The model under review builds one solid part; all positions refer to its coordinate system, in mm. Round coordinates to 2 decimals unless told otherwise and drop trailing zeros. Loops run counter-clockwise (first coordinate to the right, second up) from the corner with the lowest first, then second, coordinate; pieces in that order, holes last. Notation, with made-up numbers: M -38,63.5 L 10,63.5 A34 ccw 10,101.5 Z; hole C 29,67.5 d11. An arc over 180 degrees is marked long. Return JSON: item names as keys, results as strings. Group by question number.
Q1. Clearance check with a flat-ended pin moving along its axis: pin 1 Ø7 at (x, y) = (8.255, 17.78) entering from +Z. State where the tip first meets the part, or that it passes through.
Q2. To check wall thickness, follow line 1 along Y through (x, z) = (7, 0.45); line 2 along Y through (x, z) = (8.5, 0.75); line 3 along X through (y, z) = (16.5, 0.45). State the ranges of each line that lie inside material, in increasing order.
Q3. Consider section A-A (z = 0.75). State the section outline as (x, y) points (3 decimals), and give its area (3 significant figures).
Q4. Consider section D-D (x = 22). State the section outline as (y, z) points.
Q5. Draft analysis for pull direction Y (two halves, no side actions). For faces 1 (the face through (19, 0, 1)), 2 (the face through (0, 18, 1)), 3 (the face through (9.412, 19.595, 0.783)), 4 (the face through (9.25, 5.71, 0.78)), state which applies: pulls with the +Y half, pulls with the -Y half, needs draft (parallel to the pull), parting line crosses it, or undercut.
Q6. Consider section B-B (y = 7.62). State the section outline as (x, z) points, and give its area (3 significant figures).
Q7. Consider section C-C (y = 12.7). State the section outline as (x, z) points.
from build123d import *

# Parameters (mm, degrees)
SKETCH1_W           = 16.51
SKETCH1_H           = 25.4
SKETCH1_R           = 2.15265
SKETCH1_W_2         = 21.59
SKETCH1_R_2         = 3.2639
BOSS_EXTRUDE1_DEPTH = 1.5875


with BuildPart() as part:
    # Sketch1 → Boss-Extrude1 (new body)
    # profile 1 of 4: a face of its own
    with BuildSketch(Plane.XY):
        Polygon((0, 35.56), (0, 25.4), (16.51, 25.4), (38.1, 25.4), (38.1, 35.56), align=None)
    # profile 2 of 4: a face of its own
    with BuildSketch(Plane.XY):
        with Locations((8.255, 12.7)):
            Rectangle(SKETCH1_W, SKETCH1_H)
        with Locations((8.255, 7.62)):
            Circle(SKETCH1_R, mode=Mode.SUBTRACT)
        with Locations((8.255, 17.78)):
            Circle(SKETCH1_R, mode=Mode.SUBTRACT)
    # profile 3 of 4: a face of its own
    with BuildSketch(Plane.XY):
        with Locations((27.305, 12.7)):
            Rectangle(SKETCH1_W_2, SKETCH1_H)
        with Locations((27.305, 12.7)):
            Circle(SKETCH1_R_2, mode=Mode.SUBTRACT)
    # profile 4 of 4: a face of its own
    with BuildSketch(Plane.XY):
        Polygon((38.1, 38.34043763), (38.1, 35.56), (0, 35.56), align=None)
    extrude(amount=BOSS_EXTRUDE1_DEPTH)


solid = part.part
Values:
{
 "1": {"pin 1": "stops at z = 1.59"},
 "2": {"line 1": "y = 0 to 5.87, 9.37 to 16.03, 19.53 to 36.07", "line 2": "y = 0 to 5.48, 9.76 to 15.64, 19.92 to 36.18", "line 3": "x = 0 to 6.52, 9.99 to 38.1"},
 "3": {"outline": "M 0,0 L 38.1,0 L 38.1,38.34 L 0,35.56 Z; hole C 8.255,7.62 d4.305; hole C 8.255,17.78 d4.305; hole C 27.305,12.7 d6.528", "area": "1,350 mm2"},
 "4": {"outline": "M 0,0 L 37.17,0 L 37.17,1.59 L 0,1.59 Z"},
 "5": {"face 1": "pulls with the -Y half", "face 2": "needs draft", "face 3": "undercut", "face 4": "undercut"},
 "6": {"outline": "M 0,0 L 6.1,0 L 6.1,1.59 L 0,1.59 Z; M 10.41,0 L 38.1,0 L 38.1,1.59 L 10.41,1.59 Z", "area": "53.6 mm2"},
 "7": {"outline": "M 0,0 L 24.04,0 L 24.04,1.59 L 0,1.59 Z; M 30.57,0 L 38.1,0 L 38.1,1.59 L 30.57,1.59 Z"}
}
